Work out the finished part from the listing and answer in its coordinate system (mm). A direction names the side the tool comes from. Give positions to 0.01 mm unless a question says otherwise; leave off trailing zeros. Write each loop counter-clockwise with the first axis right and the second up, starting at its lowest first coordinate (ties: lowest second). Pieces come first, ordered by that corner, then holes.
1) Find section D-D (x = 4.25). Determine the outline of the cut face in (y, z).
2) Find section B-B (z = 1.75). Determine the outline of the cut face in (x, y).
3) A tool of negligible diameter and unlimited length cuts with its end or side. For faces 1 (the face through (-3.162, -0.5, 0)), 2 (the face through (3, -3, 1)), 3 (the face through (-0.5, -0.965, -3.4)), from which of +Z, -Z, +X, -X, +Y, -Y can it reach the whole face along a straight path? Write none if from no direction.
4) Straight lines are drawn through the part: probe 1 along Z at (x, y) = (0, -4); probe 2 along X at (y, z) = (-4.2, 0.75); probe 3 along Z at (x, y) = (1.5, -4.4). For each, find the intervals that lie inside material, in ascending order.
5) Given pin 1 Ø4.5 at (x, z) = (0, 0) entering from -Y; pin 2 Ø1.5 at (x, y) = (-3.5, -4) entering from +Z; pin 3 Ø0.8 at (y, z) = (-0.5, 0) entering from -X; pin 4 Ø1.5 at (x, y) = (-2, -2.5) entering from +Z, each flat-ended and moving along its own axis, determine where each tip first touches the part or whether it passes through.
6) Determine the mould class of faces 4 (the face through (5.918, -0.5, 3.2)), 5 (the face through (-0.1, -0.5, 3.759)), 6 (the face through (-4.56, -0.489, -2.453)) for opening direction Z: pulls with the +Z half, pulls with the -Z half, needs draft (parallel to the pull), parting line crosses it, or undercut.
7) Find section A-A (x = 0). Determine the outline of the cut face in (y, z), plus the area to 3 significant figures.
8) Find section C-C (y = -2.65). Determine the outline of the cut face in (x, z).
```python
from build123d import *

# Parameters (mm, degrees)
F0_W     = 11.8364
F0_H     = 7.5184
F1_DEPTH = 0.9652
F2_R     = 3.1623
F3_DEPTH = 4.1148
F4_R     = 1.9685
F5_DEPTH = 5.081
F7_DEPTH = 0.9662


with BuildPart() as f1:
    # F0 (on Front) → F1 (new body)
    with BuildSketch(Plane.XZ):
        Rectangle(F0_W, F0_H)
    extrude(amount=F1_DEPTH)

    # F2 (on face) → F3 (join)
    with BuildSketch(Plane.XZ.offset(0.9652)):
        Circle(F2_R)
    extrude(amount=F3_DEPTH)

    # F4 (on face) → F5 (cut, through all)
    with BuildSketch(Plane.XZ.offset(5.08)):
        Circle(F4_R)
    extrude(amount=-F5_DEPTH, mode=Mode.SUBTRACT)

    # F6 (on face) → F7 (cut, through all)
    with BuildSketch(Plane.XZ.offset(0.9652)):
        Polygon((-3.1623, -2.286), (-3.1623, 0), (-3.1623, 2.286), (-5.9182, 2.6162), (-5.9182, -2.6162), align=None)
        Polygon((3.1623, 2.286), (3.1623, 0), (3.1623, -2.286), (5.9182, -2.6162), (5.9182, 2.6162), align=None)
    extrude(amount=-F7_DEPTH, mode=Mode.SUBTRACT)


solid = f1.part
```
Results:
1. outline: (-0.97, -3.76) - (0, -3.76) - (0, -2.42) - (-0.97, -2.42) - close; (-0.97, 2.42) - (0, 2.42) - (0, 3.76) - (-0.97, 3.76) - close
2. outline: (-3.16, -0.97) - (-2.63, -0.97) - (-2.63, -5.08) - (-0.9, -5.08) - (-0.9, 0) - (-3.16, 0) - close; (0.9, -5.08) - (2.63, -5.08) - (2.63, -0.97) - (3.16, -0.97) - (3.16, 0) - (0.9, 0) - close
3. face 1: -X, +Y, -Y
3. face 2: -Y
3. face 3: -Z, -Y
4. probe 1: z = -3.16 to -1.97, 1.97 to 3.16
4. probe 2: x = -3.07 to -1.82, 1.82 to 3.07
4. probe 3: z = -2.78 to -1.27, 1.27 to 2.78
5. pin 1: stops at y = -5.08
5. pin 2: stops at z = 1.56
5. pin 3: stops at x = -3.16
5. pin 4: stops at z = 2.9
6. face 4: needs draft
6. face 5: pulls with the +Z half
6. face 6: undercut
7. outline: (-5.08, -3.16) - (-0.97, -3.16) - (-0.97, -3.76) - (0, -3.76) - (0, -1.97) - (-5.08, -1.97) - close; (-5.08, 1.97) - (0, 1.97) - (0, 3.76) - (-0.97, 3.76) - (-0.97, 3.16) - (-5.08, 3.16) - close
7. area: 13.3 mm2
8. outline: circle Ø6.32 at (0, 0); hole circle Ø3.94 at (0, 0)
